For this review, use the dimensioned drawing (mm, ordinates from the lowest corner) and the shaded views. Give positions to 0.01 mm unless a question says otherwise; leave off trailing zeros. Loops run counter-clockwise (first coordinate to the right, second up) from the corner with the lowest first, then second, coordinate; pieces in that order, holes last. Notation, with made-up numbers: (17.25, 28) -> (31.25, 28) arc R4 cw to (31.25, 35) -> close; hole circle Ø2 at (11.5, 85). An arc over 180 degrees is marked (long way). Write each question's results on one line, items separated by ' | '. Start each with the question number.
Q1. We need section A-A (y = 2.35). Write out the cut boundary in (x, z), plus the area to 3 significant figures.
Q2. We need section B-B (z = 78.5). Write out the cut boundary in (x, y), plus the area to 3 significant figures.
Q3. Insertion check: pin 1 Ø0.9 at (x, y) = (83.5, 2) entering from -Z; pin 2 Ø1.5 at (y, z) = (2, 3.5) entering from +X; pin 3 Ø1 at (y, z) = (0.5, 78) entering from +X. Each pin has a flat end and moves straight along its axis. Give the tip position at first contact, or say it passes through.
Q4. We need section C-C (x = 67). Write out the cut boundary in (y, z).
Q5. Wall thickness on L1, parallel to Z at x = 67, y = 2.05; L2, parallel to X at y = 1.75, z = 72.5: over which ranges is each line inside the solid? List them lowest first. Write a range as [from, to].
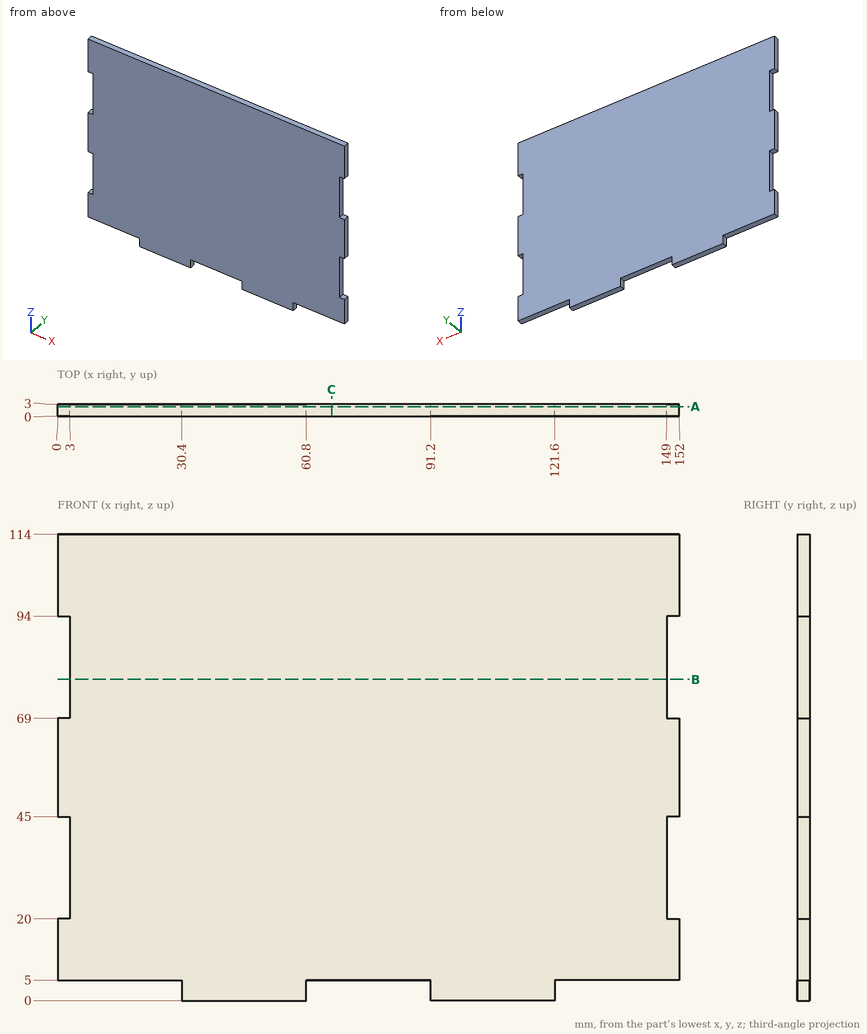
Output:
1) outline: (0, 5) -> (30.4, 5) -> (30.4, 0) -> (60.8, 0) -> (60.8, 5) -> (91.2, 5) -> (91.2, 0) -> (121.6, 0) -> (121.6, 5) -> (152, 5) -> (152, 20) -> (149, 20) -> (149, 45) -> (152, 45) -> (152, 69) -> (149, 69) -> (149, 94) -> (152, 94) -> (152, 114) -> (0, 114) -> (0, 94) -> (3, 94) -> (3, 69) -> (0, 69) -> (0, 45) -> (3, 45) -> (3, 20) -> (0, 20) -> close | area: 16,600 mm2
2) outline: (3, 0) -> (149, 0) -> (149, 3) -> (3, 3) -> close | area: 438 mm2
3) pin 1: z = 5 | pin 2: x = 121.6 | pin 3: x = 149
4) outline: (0, 5) -> (3, 5) -> (3, 114) -> (0, 114) -> close
5) L1: [5, 114] | L2: [3, 149]
